```python
from build123d import *

# Parameters (mm, degrees)
F0_W     = 85
F0_H     = 9
F0_R     = 1.5
F1_DEPTH = 2
F2_R     = 4
F3_SIZE  = 1.87


with BuildPart() as f1:
    # F0 (on Front) → F1 (new body)
    with BuildSketch(Plane.XZ):
        Rectangle(F0_W, F0_H)
        with Locations((-38, 0)):
            Circle(F0_R, mode=Mode.SUBTRACT)
        Circle(F0_R, mode=Mode.SUBTRACT)
        with Locations((38, 0)):
            Circle(F0_R, mode=Mode.SUBTRACT)
    extrude(amount=F1_DEPTH)

    # F2
    f2_edges = [f1.edges().sort_by_distance(p)[0] for p in [
        (-42.5, -1, 4.5),
        (-42.5, -1, -4.5),
        (42.5, -1, -4.5),
        (42.5, -1, 4.5),
    ]]
    fillet(f2_edges, radius=F2_R)

    # F3
    f3_edges = [f1.edges().sort_by_distance(p)[0] for p in [
        (-39.5, -2, 0),
        (36.5, 0, 0),
    ]]
    chamfer(f3_edges, length=F3_SIZE)


solid = f1.part
```
Part model, mm, in its own coordinate system. Round coordinates to 2 decimals unless told otherwise and drop trailing zeros. Write each loop counter-clockwise with the first axis right and the second up, starting at its lowest first coordinate (ties: lowest second). Pieces come first, ordered by that corner, then holes.
Item 1: Cut at A-A, the plane y = -0.75. Give the cut face in (x, z).
Results:
outline: (-42.5, -0.5) arc R4 ccw to (-38.5, -4.5) - (38.5, -4.5) arc R4 ccw to (42.5, -0.5) - (42.5, 0.5) arc R4 ccw to (38.5, 4.5) - (-38.5, 4.5) arc R4 ccw to (-42.5, 0.5) - close; hole circle Ø4.24 at (-38, 0); hole circle Ø3 at (0, 0); hole circle Ø5.24 at (38, 0)
Item 2: Cut at B-B, the plane x = 0. Give the cut face in (y, z), plus the area to 3 significant figures.
Results:
outline: (-2, -4.5) - (0, -4.5) - (0, -1.5) - (-2, -1.5) - close; (-2, 1.5) - (0, 1.5) - (0, 4.5) - (-2, 4.5) - close
area: 12.0 mm2
Item 3: Two-plate mould, pull along Z, no slides. Class faces 1 (the cylindrical face through (41.297, -1.014, 3.359)), 2 (the flat face through (-1, -1, -4.5)), 3 (the cylindrical face through (-1.5, -0.99, 0.07)): +Z half, -Z half, draft (parallel to the pull), parting line (faces both ways), or undercut.
Results:
face 1: +Z half
face 2: -Z half
face 3: undercut
Item 4: Drop a flat-ended pin along its axis: pin 1 Ø5 at (x, z) = (-38, 0) entering from +Y. Give the stop position or say it passes through.
Results:
pin 1: stops at y = 0
Item 5: Probe L1, parallel to Z at x = 0, y = -0.95; L2, parallel to X at y = -0.8, z = -0.5; L3, parallel to X at y = -0.6, z = 1. List the from-to ranges inside material, lowest first.
Results:
L1: z = -4.5 to -1.5, 1.5 to 4.5
L2: x = -42.5 to -40.11, -35.89 to -1.41, 1.41 to 35.48, 40.52 to 42.5
L3: x = -42.47 to -39.7, -36.3 to -1.12, 1.12 to 35.42, 40.58 to 42.47
